The model under review builds one solid part; all positions refer to its coordinate system, in mm. A direction names the side the tool comes from. Coordinates: 2 decimals unless noted, no trailing zeros. Loops run counter-clockwise (first coordinate to the right, second up) from the corner with the lowest first, then second, coordinate; pieces in that order, holes last. Notation, with made-up numbers: M -14,10 L 5,10 A26 cw 5,34 Z; hole C -10,-29.75 d6. An arc over 180 degrees is marked long. Return JSON: item names as keys, results as strings.
```python
from build123d import *

# Parameters (mm, degrees)
SKETCH1_W               = 77.514562268
SKETCH1_H               = 12
BOSS_EXTRUDE1_DEPTH     = 1.47955
CUT_EXTRUDE1_DEPTH      = 93.316205492
CUT_EXTRUDE1_DEPTH_BACK = 93.316205492
SKETCH3_R               = 0.92964


with BuildPart() as part:
    # Sketch1 → Boss-Extrude1 (new, symmetric)
    with BuildSketch(Plane.XY):
        with Locations((-53.29272171, -0.35)):
            Rectangle(SKETCH1_W, SKETCH1_H)
    extrude(amount=BOSS_EXTRUDE1_DEPTH, both=True)

    # Sketch3 → Cut-Extrude1 (cut, two sides: drawn at the far end of the back side and taken through both)
    with BuildSketch(Plane(origin=(0, 0, -1.47955), x_dir=(-1, 0, 0), z_dir=(0, 0, -1)).offset(-CUT_EXTRUDE1_DEPTH_BACK)):
        with Locations((18.000000576, 2.65)):
            Circle(SKETCH3_R)
        with Locations((90.00000288, 2.65)):
            Circle(SKETCH3_R)
        with BuildLine():
            Line((26.1081454, 2.65), (26.1081454, 5.65))
            Line((26.1081454, 5.65), (27.9674254, 5.65))
            Line((27.9674254, 5.65), (27.9674254, 2.65))
            ThreePointArc((27.9674254, 2.65), (27.0377854, 1.72036), (26.1081454, 2.65))
        make_face()
        with BuildLine():
            Line((35.09872244, 2.65), (35.09872244, 5.65))
            Line((35.09872244, 5.65), (36.95800244, 5.65))
            Line((36.95800244, 5.65), (36.95800244, 2.65))
            ThreePointArc((36.95800244, 2.65), (36.02836244, 1.72036), (35.09872244, 2.65))
        make_face()
        with BuildLine():
            Line((44.093057534, 2.65), (44.093057534, 5.65))
            Line((44.093057534, 5.65), (45.952337534, 5.65))
            Line((45.952337534, 5.65), (45.952337534, 2.65))
            ThreePointArc((45.952337534, 2.65), (45.022697534, 1.72036), (44.093057534, 2.65))
        make_face()
        with BuildLine():
            Line((53.089277696, 2.65), (53.089277696, 5.65))
            Line((53.089277696, 5.65), (54.948557696, 5.65))
            Line((54.948557696, 5.65), (54.948557696, 2.65))
            ThreePointArc((54.948557696, 2.65), (54.018917696, 1.72036), (53.089277696, 2.65))
        make_face()
        with BuildLine():
            Line((62.086576691, 2.65), (62.086576691, 5.65))
            Line((62.086576691, 5.65), (63.945856691, 5.65))
            Line((63.945856691, 5.65), (63.945856691, 2.65))
            ThreePointArc((63.945856691, 2.65), (63.016216691, 1.72036), (62.086576691, 2.65))
        make_face()
        with BuildLine():
            Line((71.084550518, 2.65), (71.084550518, 5.65))
            Line((71.084550518, 5.65), (72.943830518, 5.65))
            Line((72.943830518, 5.65), (72.943830518, 2.65))
            ThreePointArc((72.943830518, 2.65), (72.014190518, 1.72036), (71.084550518, 2.65))
        make_face()
        with BuildLine():
            Line((80.08297445, 2.65), (80.08297445, 5.65))
            Line((80.08297445, 5.65), (81.94225445, 5.65))
            Line((81.94225445, 5.65), (81.94225445, 2.65))
            ThreePointArc((81.94225445, 2.65), (81.01261445, 1.72036), (80.08297445, 2.65))
        make_face()
    extrude(amount=CUT_EXTRUDE1_DEPTH + CUT_EXTRUDE1_DEPTH_BACK, mode=Mode.SUBTRACT)


solid = part.part
```
1. Add section A-A on x = -18. Give the boundary of the cut face in (y, z).
Check values:
{"outline": "M -6.35,-1.48 L 1.72,-1.48 L 1.72,1.48 L -6.35,1.48 Z; M 3.58,-1.48 L 5.65,-1.48 L 5.65,1.48 L 3.58,1.48 Z"}
2. Add section C-C on x = -54. Give the boundary of the cut face in (y, z), plus the area to 3 significant figures.
Check values:
{"outline": "M -6.35,-1.48 L 1.72,-1.48 L 1.72,1.48 L -6.35,1.48 Z", "area": "23.9 mm²"}
3. Insertion check: pin 1 Ø2.5 at (x, y) = (-18, 2.65) entering from -Z. The pin has a flat end and moves straight along its axis. Give the tip position at first contact, or say it passes through.
Check values:
{"pin 1": "z = -1.48"}
4. Machinability: for faces 4 (the face through (-68, 5.65, 0)), 5 (the face through (-54.949, 4, 0)), which of the approach directions +Z, -Z, +X, -X, +Y, -Y give a long, thin tool a straight path to every point of the face, cutting with its end or side? Answer none if there is none.
Check values:
{"face 4": "+Z, -Z, +X, -X, +Y", "face 5": "+Z, -Z, +Y"}
5. To check wall thickness, follow line 1 (Y direction, x = -18, z = -0.5); line 2 (Y direction, x = -27, z = -0.25); line 3 (Y direction, x = -44.5, z = 1). State the ranges of each line that lie inside material, in increasing order.
Check values:
{"line 1": "-6.35 to 1.72, 3.58 to 5.65", "line 2": "-6.35 to 1.72", "line 3": "-6.35 to 1.88"}
6. The part is to be moulded in two halves that separate along X. For faces 1 (the face through (-20, 5.65, 0)), 2 (the face through (-89.315, 3.278, 0.021)), 3 (the face through (-14.535, 0, 0)), say which applies: released by +X, released by -X, zero draft, split by the parting line, or undercut.
Check values:
{"face 1": "zero draft", "face 2": "undercut", "face 3": "released by +X"}
7. Add section B-B on z = 0.05. State how many separate pieces and enclosed holes the cut face has, plus the area to 3 significant figures.
Check values:
{"separate pieces": "1", "enclosed holes": "2", "area": "876 mm²"}
